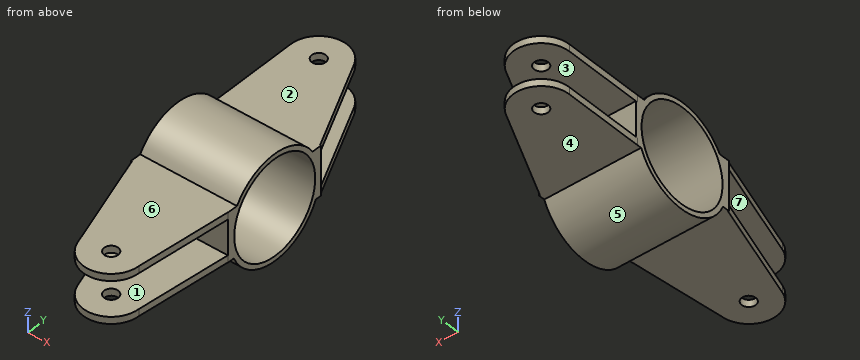
from build123d import *

# Parameters (mm, degrees)
SKETCH1_R             = 37.5
SKETCH1_R_2           = 34
BOSS_EXTRUDE1_DEPTH   = 35
BOSS_EXTRUDE2_START   = 15
SKETCH2_R             = 5
BOSS_EXTRUDE2_DEPTH   = 5
BOSS_EXTRUDE2_2_DEPTH = 5
BOSS_EXTRUDE3_START   = -15
SKETCH2_2_R           = 5
BOSS_EXTRUDE3_DEPTH   = 5
BOSS_EXTRUDE3_2_DEPTH = 5
BOSS_EXTRUDE4_DEPTH   = 70
BOSS_EXTRUDE5_START   = -70
BOSS_EXTRUDE5_DEPTH   = 70


with BuildPart() as part:
    # Sketch1 → Boss-Extrude1 (new, symmetric)
    with BuildSketch(Plane(origin=(0, 0, 0), x_dir=(0, 0, -1), z_dir=(1, 0, 0))):
        Circle(SKETCH1_R)
        Circle(SKETCH1_R_2, mode=Mode.SUBTRACT)
    extrude(amount=BOSS_EXTRUDE1_DEPTH, both=True)



with BuildPart() as body_2:
    # Sketch2 → Boss-Extrude2 (new body)
    with BuildSketch(Plane.XY.offset(BOSS_EXTRUDE2_START)):
        with BuildLine():
            Line((-36.046360502, 95.880386994), (-35, 37.5))
            Line((-35, 37.5), (35, 37.5))
            Line((35, 37.5), (1.90425986, 105.037379634))
            ThreePointArc((1.90425986, 105.037379634), (-20.743145305, 115.677666176), (-36.046360502, 95.880386994))
        make_face()
        with Locations((-16.052783226, 96.238734902)):
            Circle(SKETCH2_R, mode=Mode.SUBTRACT)
    extrude(amount=BOSS_EXTRUDE2_DEPTH)


with BuildPart() as body_3:
    # Sketch2 → Boss-Extrude2 2 (new body)
    with BuildSketch(Plane.XY.offset(BOSS_EXTRUDE2_START)):
        with BuildLine():
            Line((-35, -37.5), (35, -37.5))
            Line((35, -37.5), (28.89703955, -106.961265098))
            ThreePointArc((28.89703955, -106.961265098), (12.060917272, -126.709426475), (-10.101948226, -113.209341881))
            Line((-10.101948226, -113.209341881), (-35, -37.5))
        make_face()
        with Locations((8.89703955, -106.961265098)):
            Circle(SKETCH2_R, mode=Mode.SUBTRACT)
    extrude(amount=BOSS_EXTRUDE2_2_DEPTH)


with BuildPart() as body_4:
    # Sketch2<2> → Boss-Extrude3 (new body)
    with BuildSketch(Plane.XY.offset(BOSS_EXTRUDE3_START)):
        with BuildLine():
            Line((-36.046360502, 95.880386994), (-35, 37.5))
            Line((-35, 37.5), (35, 37.5))
            Line((35, 37.5), (1.90425986, 105.037379634))
            ThreePointArc((1.90425986, 105.037379634), (-20.743145305, 115.677666176), (-36.046360502, 95.880386994))
        make_face()
        with Locations((-16.052783226, 96.238734902)):
            Circle(SKETCH2_2_R, mode=Mode.SUBTRACT)
    extrude(amount=BOSS_EXTRUDE3_DEPTH)


with BuildPart() as body_5:
    # Sketch2<2> → Boss-Extrude3 2 (new body)
    with BuildSketch(Plane.XY.offset(BOSS_EXTRUDE3_START)):
        with BuildLine():
            Line((-35, -37.5), (35, -37.5))
            Line((35, -37.5), (28.89703955, -106.961265098))
            ThreePointArc((28.89703955, -106.961265098), (12.060917272, -126.709426475), (-10.101948226, -113.209341881))
            Line((-10.101948226, -113.209341881), (-35, -37.5))
        make_face()
        with Locations((8.89703955, -106.961265098)):
            Circle(SKETCH2_2_R, mode=Mode.SUBTRACT)
    extrude(amount=BOSS_EXTRUDE3_2_DEPTH)


with BuildPart() as part_1:
    add(part.part)

    add(body_2.part)  # Boss-Extrude4 merges body 2

    add(body_4.part)  # Boss-Extrude4 merges body 4
    # Sketch3 → Boss-Extrude4 (add)
    with BuildSketch(Plane(origin=(35, 0, 0), x_dir=(0, 0, -1), z_dir=(1, 0, 0))):
        with BuildLine():
            Line((-20, 37.5), (-20, 31.721443851))
            ThreePointArc((-20, 31.721443851), (-2.828923646, 37.393143636), (15, 34.369317712))
            Line((15, 34.369317712), (15, 37.5))
            Line((15, 37.5), (15, 38.756727822))
            Line((15, 38.756727822), (-20, 38.756727822))
            Line((-20, 38.756727822), (-20, 37.5))
        make_face()
    extrude(amount=-BOSS_EXTRUDE4_DEPTH)


    add(body_3.part)  # Boss-Extrude5 merges body 3

    add(body_5.part)  # Boss-Extrude5 merges body 5
    # Sketch4 → Boss-Extrude5 (add)
    with BuildSketch(Plane.ZY.offset(35).offset(BOSS_EXTRUDE5_START)):
        with BuildLine():
            Line((-15, -39.232593617), (20, -39.232593617))
            Line((20, -39.232593617), (20, -31.721443851))
            ThreePointArc((20, -31.721443851), (2.828923646, -37.393143636), (-15, -34.369317712))
            Line((-15, -34.369317712), (-15, -39.232593617))
        make_face()
    extrude(amount=BOSS_EXTRUDE5_DEPTH)


solid = part_1.part
For this review, take the finished solid that the model builds, in its own axes (mm). Face numbers are marked on the shaded views. A direction names the side the tool comes from. Give positions to 0.01 mm unless a question says otherwise; leave off trailing zeros. Loops run counter-clockwise (first coordinate to the right, second up) from the corner with the lowest first, then second, coordinate; pieces in that order, holes last. Notation, with made-up numbers: M 0.5,-28.5 L 51.5,-28.5 A24 ccw 51.5,7.5 Z; hole C 88,34 d5. An arc over 180 degrees is marked long. Put each result on its own line as item: value. Start each with the question number.
(1) Wall thickness on L1, parallel to Z at x = 19.5, y = -46; L2, parallel to Y at x = 0, z = 0; L3, parallel to Y at x = 25.5, z = 21.5: over which ranges is each line inside the solid? List them lowest first.
(2) The part is to be moulded in two halves that separate along Z. For the marked faces 5, 6 and 7, say which applies: +Z half, -Z half, draft (parallel to the pull), parting line (faces both ways), or undercut.
(3) Add section A-A, the plane y = 0. Write out the cut boundary in (x, z), then the cut area to 3 significant figures.
(4) Add section D-D, the plane x = -32. Write out the cut boundary in (y, z), then the cut area to 3 significant figures.
(5) For pin 1 (1 mm diameter, centred on x = -9.5, z = 28.5, fed in from +Y); pin 2 (16 mm diameter, centred on x = 8.9, y = -106.96, fed in from -Z); pin 3 (10 mm diameter, centred on y = 37.5, z = -4, fed in from -X), all flat-tipped, find the tip position at first contact; note any pin that passes through.
(6) Add section C-C, the plane z = 12. Write out the cut boundary in (x, y), then the cut area to 3 significant figures.
(7) Add section B-B, the plane x = -18.5. Write out the cut boundary in (y, z), then the cut area to 3 significant figures.
(8) Machinability: for the marked faces 1, 2, 3 and 4, which of the approach directions +Z, -Z, +X, -X, +Y, -Y give a long, thin tool a straight path to every point of the face, cutting with its end or side? Answer none if there is none.
Result:
1. L1: z = -15 to -10, 15 to 20
1. L2: y = -39.23 to -34, 34 to 38.76
1. L3: y = -30.72 to -26.34, 26.34 to 30.72
2. face 5: -Z half
2. face 6: +Z half
2. face 7: undercut
3. outline: M -35,-37.5 L 35,-37.5 L 35,-34 L -35,-34 Z; M -35,34 L 35,34 L 35,37.5 L -35,37.5 Z
3. area: 490 mm^2
4. outline: M -46.62,-15 L -34.37,-15 A37.5 ccw 34.37,-15 L 108.3,-15 L 108.3,-10 L 38.76,-10 L 38.76,15 L 108.3,15 L 108.3,20 L 31.72,20 A37.5 ccw -31.72,20 L -46.62,20 L -46.62,15 L -39.23,15 L -39.23,-10 L -46.62,-10 Z; hole C 0,0 d68
4. area: 1,770 mm^2
5. pin 1: stops at y = 24.94
5. pin 2: stops at z = -15
5. pin 3: stops at x = -35
6. outline: M -35,-39.23 L 35,-39.23 L 35,-31.81 L -35,-31.81 Z; M -35,31.81 L 35,31.81 L 35,38.76 L -35,38.76 Z
6. area: 1,010 mm^2
7. outline: M -87.67,-15 L -34.37,-15 A37.5 ccw 34.37,-15 L 91.88,-15 L 91.88,-10 L 38.76,-10 L 38.76,15 L 91.88,15 L 91.88,20 L 31.72,20 A37.5 ccw -31.72,20 L -87.67,20 L -87.67,15 L -39.23,15 L -39.23,-10 L -87.67,-10 Z; M 100.6,-15 L 116.09,-15 L 116.09,-10 L 100.6,-10 Z; M 100.6,15 L 116.09,15 L 116.09,20 L 100.6,20 Z; hole C 0,0 d68
7. area: 2,170 mm^2
8. face 1: +X, -X, -Y
8. face 2: +Z, +X, -X, +Y
8. face 3: +X, -X, +Y
8. face 4: -Z, +X, -X, +Y
